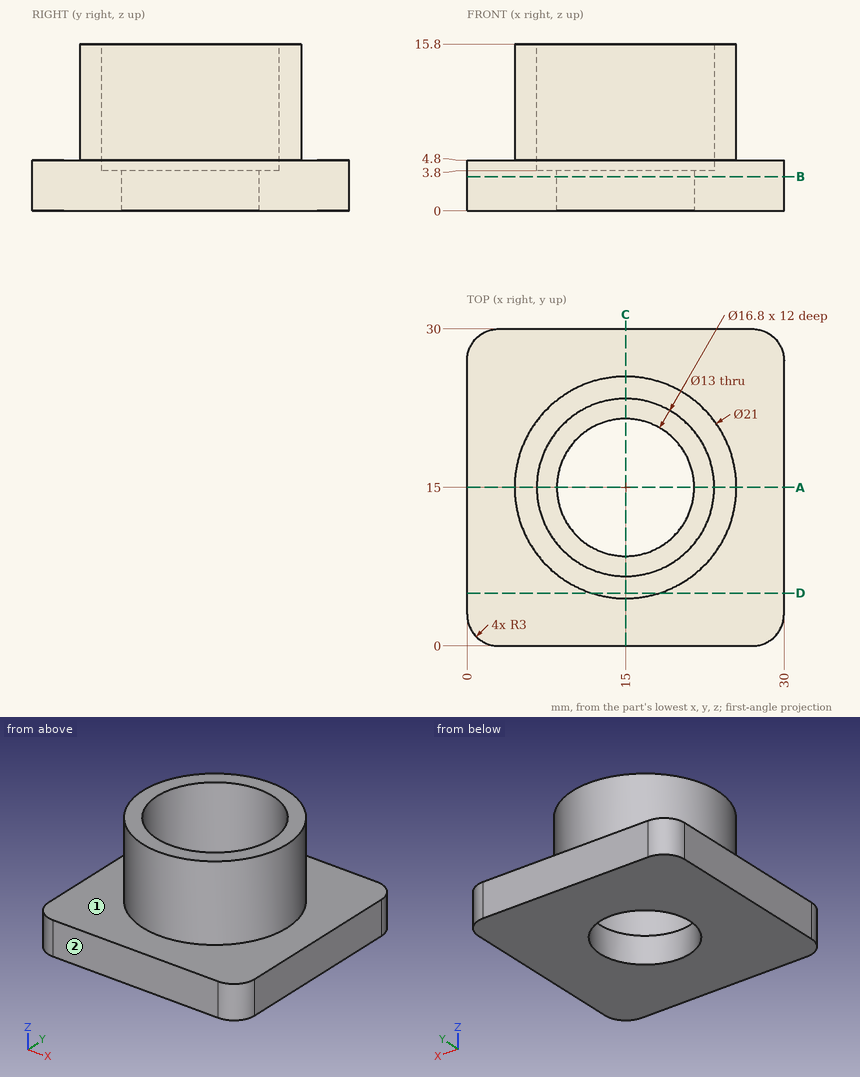
Geometry check sheet. Reference: drawing and pictorial views, mm from the part's lowest x, y, z. A direction names the side the tool comes from. Round coordinates to 2 decimals unless told otherwise and drop trailing zeros. Order: outer loops, then holes, each group sorted by start corner. A loop starts at its lowest first (then second) coordinate and runs counter-clockwise, first axis right, second up. Notation, with made-up numbers: M -21.75,33.25 L -10.75,33.25 A20 cw -10.75,47.25 Z; hole C -5,10.25 d7. An arc over 180 degrees is marked long. Answer in a Markdown table with one row per item.
(1) Go/stop test with flat-tipped pins: P1, Ø4, axis at x = 10, y = 13, coming from the +Z side; P2, Ø1, axis at y = 8.5, z = 9, coming from the -X side; P3, Ø6, axis at x = 24.5, z = 14, coming from the -Y side. Record where each tip stops, or that it passes through.
Responses:
| item | result |
|---|---|
| P1 | stops at z = 3.8 |
| P2 | stops at x = 6.38 |
| P3 | stops at y = 6.75 |
(2) Sectioned sample at B-B, the plane z = 3.25. Record the cut outline in (x, y), and give its area (3 significant figures).
Responses:
| item | result |
|---|---|
| outline | M 0,3 A3 ccw 3,0 L 27,0 A3 ccw 30,3 L 30,27 A3 ccw 27,30 L 3,30 A3 ccw 0,27 Z; hole C 15,15 d13 |
| area | 760 mm² |
(3) Sectioned sample at A-A, the plane y = 15. Record the cut outline in (x, z), and give its area (3 significant figures).
Responses:
| item | result |
|---|---|
| outline | M 0,0 L 8.5,0 L 8.5,3.8 L 6.6,3.8 L 6.6,15.8 L 4.5,15.8 L 4.5,4.8 L 0,4.8 Z; M 21.5,0 L 30,0 L 30,4.8 L 25.5,4.8 L 25.5,15.8 L 23.4,15.8 L 23.4,3.8 L 21.5,3.8 Z |
| area | 124 mm² |
(4) Sectioned sample at D-D, the plane y = 5. Record the cut outline in (x, z).
Responses:
| item | result |
|---|---|
| outline | M 0,0 L 30,0 L 30,4.8 L 18.2,4.8 L 18.2,15.8 L 11.8,15.8 L 11.8,4.8 L 0,4.8 Z |
(5) Tool access check on the marked faces 1 and 2. Record the directions out of +Z, -Z, +X, -X, +Y, -Y that give a thin tool (end or side, any length) a straight path to the whole face; none if there is none.
Responses:
| item | result |
|---|---|
| face 1 | +Z |
| face 2 | +Z, -Z, +X, -X, -Y |
(6) Scan lines: probe 1 along Y at (x, z) = (15, 12); probe 2 along Y at (x, z) = (15, 1); probe 3 along Z at (x, y) = (19.75, 20.75). Record each from-to range of solid material in increasing order. Write a range as from..to.
Responses:
| item | result |
|---|---|
| probe 1 | y = 4.5..6.6, 23.4..25.5 |
| probe 2 | y = 0..8.5, 21.5..30 |
| probe 3 | z = 0..3.8 |
